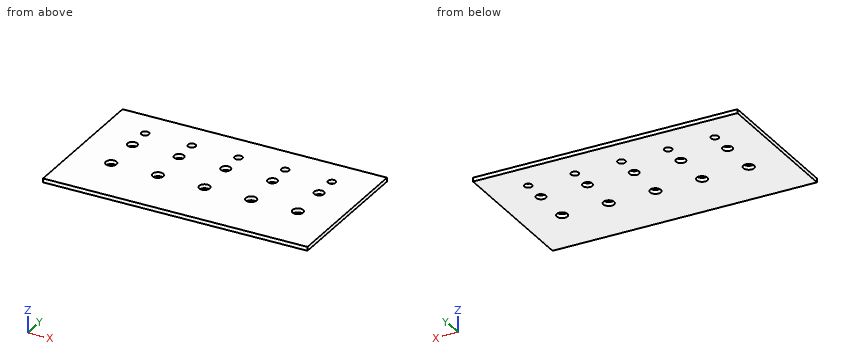
Autodesk Inventor part; units mm, degrees
ref_plane "YZ Plane" through (0, 0, 0) normal (1, 0, 0) x (0, 1, 0)
ref_plane "XZ Plane" through (0, 0, 0) normal (0, 1, 0) x (-1, 0, 0)
ref_plane "XY Plane" through (0, 0, 0) normal (0, 0, 1) x (1, 0, 0)
sketch "Sketch1" plane through (0, 0, 0) normal (0, 0, 1) x (1, 0, 0)
  line L0 (0, 0) -> (172.72, 0)
  line L1 (172.72, 0) -> (172.72, 95.25)
  line L2 (172.72, 95.25) -> (0, 95.25)
  line L3 (0, 95.25) -> (0, 0)
  dimension "d53" = 172.72
  dimension "d57" = 95.25
extrude "Extrusion1" add sketch "Sketch1" along normal blind 2.54
sketch "Sketch2" plane through (0, 0, 2.54) normal (0, 0, 1) x (1, 0, 0)
  circle A0 centre (25.4, 35.121) radius 3.5
  circle A1 centre (25.4, 60.521) radius 3.175
  line L0 (0, 95.25) -> (0, 0)
  circle A2 centre (55.88, 60.521) radius 3.175
  circle A3 centre (86.36, 60.521) radius 3.175
  circle A4 centre (116.84, 60.521) radius 3.175
  circle A5 centre (147.32, 60.521) radius 3.175
  circle A6 centre (25.4, 75.761) radius 2.5
  circle A7 centre (55.88, 75.761) radius 2.5
  circle A8 centre (86.36, 75.761) radius 2.5
  circle A9 centre (116.84, 75.761) radius 2.5
  circle A10 centre (147.32, 75.761) radius 2.5
  circle A11 centre (55.88, 35.121) radius 3.5
  circle A12 centre (86.36, 35.121) radius 3.5
  circle A13 centre (116.84, 35.121) radius 3.5
  circle A14 centre (147.32, 35.121) radius 3.5
  line L1 (172.72, 0) -> (172.72, 95.25)
  dimension "d4" = 7
  dimension "d5" = 6.35
  dimension "d8" = 25.4
  dimension "d9" = 6.35
  dimension "d10" = 6.35
  dimension "d11" = 6.35
  dimension "d12" = 6.35
  dimension "d18" = 0
  dimension "d19" = 0
  dimension "d20" = 0
  dimension "d21" = 0
  dimension "d22" = 5
  dimension "d23" = 15.24
  dimension "d24" = 0
  dimension "d25" = 5
  dimension "d26" = 5
  dimension "d27" = 5
  dimension "d28" = 5
  dimension "d29" = 15.24
  dimension "d34" = 15.24
  dimension "d35" = 15.24
  dimension "d36" = 15.24
  dimension "d37" = 7
  dimension "d38" = 7
  dimension "d39" = 7
  dimension "d40" = 7
  dimension "d41" = 30.48
  dimension "d42" = 25.4
  dimension "d43" = 30.48
  dimension "d44" = 25.4
  dimension "d45" = 30.48
  dimension "d46" = 25.4
  dimension "d47" = 30.48
  dimension "d48" = 25.4
  dimension "d49" = 30.48
  dimension "d50" = 30.48
  dimension "d51" = 30.48
  dimension "d52" = 30.48
  dimension "d58" = 30.48
  dimension "d59" = 30.48
  dimension "d60" = 30.48
  dimension "d61" = 30.48
  dimension "d62" = 0
  dimension "d63" = 25.4
extrude "Extrusion2" cut sketch "Sketch2" against normal blind 2.54
properties part number "front"
Design review of the part built by this model. Coordinates are the model's own, in mm. Coordinates: 2 decimals unless noted, no trailing zeros. Loops run counter-clockwise (first coordinate to the right, second up) from the corner with the lowest first, then second, coordinate; pieces in that order, holes last. Notation, with made-up numbers: M -22.75,66 L 14.25,66 A24 cw 14.25,97 Z; hole C 45.25,88.25 d1. An arc over 180 degrees is marked long. Answer as CSV lines item,"result".
Item 1: Add section C-C on x = 87. State the section outline as (y, z) points, plus the area to 3 significant figures.
Answer list:
outline,"M 0,0 L 31.68,0 L 31.68,2.54 L 0,2.54 Z; M 38.56,0 L 57.41,0 L 57.41,2.54 L 38.56,2.54 Z; M 63.63,0 L 73.34,0 L 73.34,2.54 L 63.63,2.54 Z; M 78.18,0 L 95.25,0 L 95.25,2.54 L 78.18,2.54 Z"
area,"196 mm²"
Item 2: For probe 1 along X at (y, z) = (76, 1.4); probe 2 along Y at (x, z) = (147.32, 0.65); probe 3 along X at (y, z) = (58.5, 1.3), list the stretches that pass through material, from the lowest coordinate up.
Answer list:
probe 1,"0 to 22.91, 27.89 to 53.39, 58.37 to 83.87, 88.85 to 114.35, 119.33 to 144.83, 149.81 to 172.72"
probe 2,"0 to 31.62, 38.62 to 57.35, 63.7 to 73.26, 78.26 to 95.25"
probe 3,"0 to 22.95, 27.85 to 53.43, 58.33 to 83.91, 88.81 to 114.39, 119.29 to 144.87, 149.77 to 172.72"
Item 3: Add section A-A on x = 116.84. State the section outline as (y, z) points.
Answer list:
outline,"M 0,0 L 31.62,0 L 31.62,2.54 L 0,2.54 Z; M 38.62,0 L 57.35,0 L 57.35,2.54 L 38.62,2.54 Z; M 63.7,0 L 73.26,0 L 73.26,2.54 L 63.7,2.54 Z; M 78.26,0 L 95.25,0 L 95.25,2.54 L 78.26,2.54 Z"
Item 4: Add section B-B on z = 1.45. Count the separate pieces of the cut face and the enclosed holes in it, plus the area to 3 significant figures.
Answer list:
separate pieces,"1"
enclosed holes,"15"
area,"16,000 mm²"
